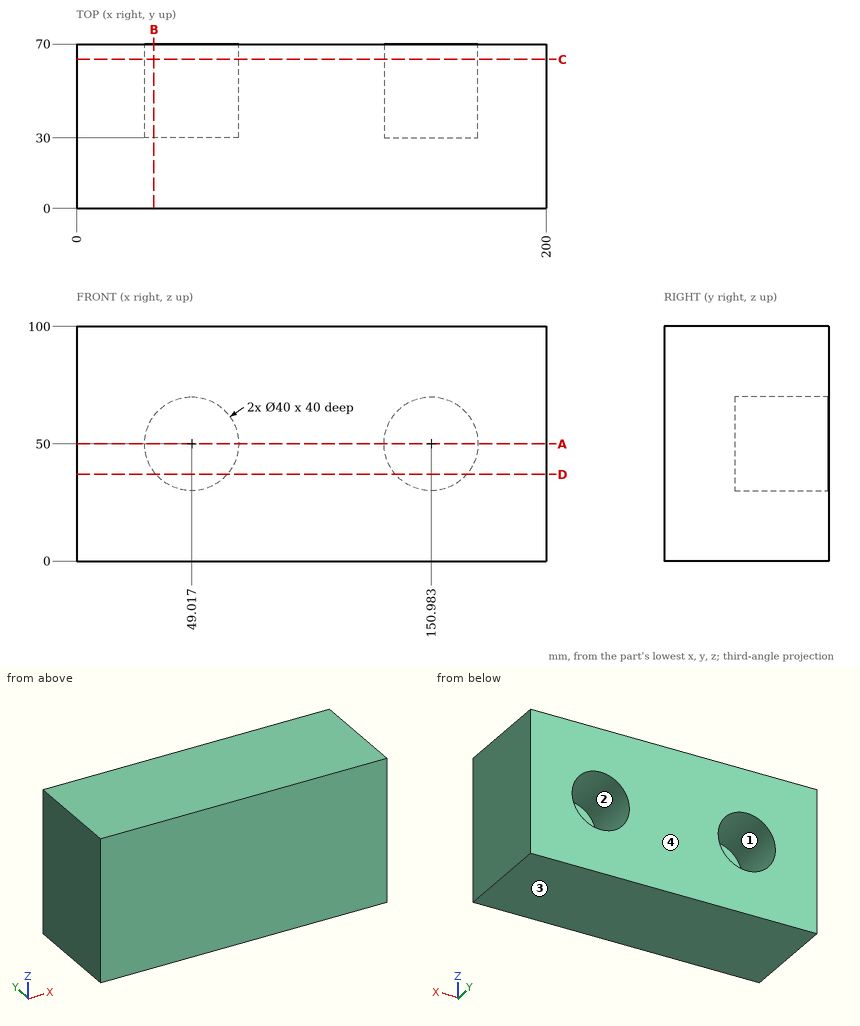
Geometry check sheet. Reference: drawing and pictorial views, mm from the part's lowest x, y, z. Coordinates: 2 decimals unless noted, no trailing zeros. Write each loop counter-clockwise with the first axis right and the second up, starting at its lowest first coordinate (ties: lowest second). Pieces come first, ordered by that corner, then holes. Notation, with made-up numbers: (-8, 65) - (37, 65) arc R20 cw to (37, 77) - close; hole circle Ø11 at (69, -27). An arc over 180 degrees is marked (long way). Write item = value, one per line.
Q1. Cross-section at B-B (x = 33). Enter the section's corners in (y, z).
Answer:
outline = (0, 0) - (70, 0) - (70, 38.02) - (30, 38.02) - (30, 61.98) - (70, 61.98) - (70, 100) - (0, 100) - close
Q2. Go/stop test with a flat-tipped pin: pin 1 Ø12 at (x, z) = (145, 55) entering from +Y. Record where the tip stops, or that it passes through.
Answer:
pin_1 = 30
Q3. Cross-section at D-D (z = 37). Enter the section's corners in (x, y).
Answer:
outline = (0, 0) - (200, 0) - (200, 70) - (166.18, 70) - (166.18, 30) - (135.78, 30) - (135.78, 70) - (64.22, 70) - (64.22, 30) - (33.82, 30) - (33.82, 70) - (0, 70) - close
Q4. Cross-section at A-A (z = 50). Enter the section's corners in (x, y).
Answer:
outline = (0, 0) - (200, 0) - (200, 70) - (170.98, 70) - (170.98, 30) - (130.98, 30) - (130.98, 70) - (69.02, 70) - (69.02, 30) - (29.02, 30) - (29.02, 70) - (0, 70) - close
Q5. Mould release check, pull along Z, two halves, no side actions. Record for the marked faces 1, 2, 3 and 4: released by +Z, released by -Z, zero draft, split by the parting line, or undercut.
Answer:
face_1 = undercut
face_2 = undercut
face_3 = released by -Z
face_4 = zero draft
Q6. Material ranges on L1, parallel to X at y = 66, z = 32.5 (1 decimal); L2, parallel to X at y = 53, z = 61.5 (1 decimal); L3, parallel to Y at x = 153.5, z = 63, recorded low to high. Write a range as from..to.
Answer:
L1 = 0..39.3, 58.7..141.3, 160.7..200
L2 = 0..32.7, 65.4..134.6, 167.3..200
L3 = 0..30
Q7. Cross-section at C-C (y = 63.5). Enter the section's corners in (x, z).
Answer:
outline = (0, 0) - (200, 0) - (200, 100) - (0, 100) - close; hole circle Ø40 at (49.02, 50); hole circle Ø40 at (150.98, 50)
